For this review, take the finished solid that the model builds, in its own axes (mm). Round coordinates to 2 decimals unless told otherwise and drop trailing zeros. Loops run counter-clockwise (first coordinate to the right, second up) from the corner with the lowest first, then second, coordinate; pieces in that order, holes last. Notation, with made-up numbers: M -10,-9.75 L 25,-9.75 A22 ccw 25,16.25 Z; hole C 76.5,40 d11. An arc over 180 degrees is marked long. One line per question, with ' | ' between items. Start each with the question number.
1) For probe 1 along Y at (x, z) = (-3, -0.4); probe 2 along Y at (x, z) = (-4.5, -1.4); probe 3 along X at (y, z) = (5.25, -0.3), list the stretches that pass through material, from the lowest coordinate up. Write a range as from..to.
2) Mouldability with a two-part tool opening along X and no side actions: class faces 1 (the face through (-5.04, 3.86, 0.02)), 2 (the face through (3.51, -6.17, -0.02)), 3 (the face through (1.6, 6.3, 1.588)) as pulls with the +X half, pulls with the -X half, needs draft (parallel to the pull), parting line crosses it, or undercut.
3) We need section A-A (x = 0). Give the boundary of the cut face in (y, z).
4) We need section B-B (z = 0.75). Give the boundary of the cut face in (x, y), and give its area (3 significant figures).
```python
from build123d import *

# Parameters (mm, degrees)
CUT_EXTRUDE1_DEPTH      = 12.357322055
CUT_EXTRUDE1_DEPTH_BACK = 12.357322055
SKETCH4_OUTSIDE_W       = 22.446
SKETCH4_OUTSIDE_H       = 22.446


with BuildPart() as part:
    # Sketch3 → Revolve1 (revolve)
    with BuildSketch(Plane(origin=(0, 0, 0), x_dir=(0, 0, -1), z_dir=(1, 0, 0)), mode=Mode.PRIVATE) as revolve1_sk:
        Polygon((-1.5875, 7.1), (-1.095597571, 7.952), (1.095597571, 7.952), (1.5875, 7.1), (1.5875, 6.35), (-1.5875, 6.35), align=None)
    revolve(revolve1_sk.sketch.rotate(Axis((0, 0, 1.5875), (0, 0, -1)), 90), axis=Axis((0, 0, 1.5875), (0, 0, -1)))

    # Sketch4 outside → Cut-Extrude1 (cut, two sides: drawn at the far end of the back side and taken through both)
    with BuildSketch(Plane.XY.offset(-CUT_EXTRUDE1_DEPTH_BACK)):
        Rectangle(SKETCH4_OUTSIDE_W, SKETCH4_OUTSIDE_H)
        Polygon((0, 8.198373822), (-7.1, 4.099186911), (-7.1, -4.099186911), (0, -8.198373822), (7.1, -4.099186911), (7.1, 4.099186911), align=None, mode=Mode.SUBTRACT)
    extrude(amount=CUT_EXTRUDE1_DEPTH + CUT_EXTRUDE1_DEPTH_BACK, mode=Mode.SUBTRACT)


solid = part.part
```
Answers below:
1) probe 1: -6.47..-5.6, 5.6..6.47 | probe 2: -5.6..-4.48, 4.48..5.6 | probe 3: -5.11..-3.57, 3.57..5.11
2) face 1: undercut | face 2: pulls with the +X half | face 3: needs draft
3) outline: M -7.95,-1.1 L -7.1,-1.59 L -6.35,-1.59 L -6.35,1.59 L -7.1,1.59 L -7.95,1.1 Z; M 6.35,-1.59 L 7.1,-1.59 L 7.95,-1.1 L 7.95,1.1 L 7.1,1.59 L 6.35,1.59 Z
4) outline: M -7.1,-3.58 A7.95 ccw -6.65,-4.36 L -0.45,-7.94 A7.95 ccw 0.45,-7.94 L 6.65,-4.36 A7.95 ccw 7.1,-3.58 L 7.1,3.58 A7.95 ccw 6.65,4.36 L 0.45,7.94 A7.95 ccw -0.45,7.94 L -6.65,4.36 A7.95 ccw -7.1,3.58 Z; hole C 0,0 d12.7 | area: 47.3 mm^2
